Input: part model. Units: mm. Frame: model coordinates. A direction names the side the tool comes from. Round coordinates to 2 decimals unless told otherwise and drop trailing zeros. Loops run counter-clockwise (first coordinate to the right, second up) from the corner with the lowest first, then second, coordinate; pieces in that order, holes last. Notation, with made-up numbers: (49, 73) - (67, 73) arc R17 cw to (67, 87) - close; hole circle Ø10 at (72, 34). An arc over 180 degrees is marked (long way). One line per question, with ' | ' between items. Start each with the question number.
Item 1: Section A-A, the plane x = -47.5. Return loops of the section in (y, z).
Item 2: Set-up query: faces 1 (the face through (-31, 21, 0)), 2 (the face through (-31.04, 15.88, -10.9)), 3 (the face through (-31.04, -10.86, 15.84)), 4 (the face through (-31.035, 9.605, 9.713)), 5 (the face through (-42.5, 3, -3)). Return all of +Z, -Z, +X, -X, +Y, -Y with unobstructed straight access to the full face (end or side cutting, diameter ignored); none if empty.
Item 3: Section B-B, the plane x = 32. Return loops of the section in (y, z), plus the area to 3 significant figures.
Item 4: Material intervals for line 1 along Z through (x, y) = (-27.5, 0); line 2 along Z through (x, y) = (-33, 11.5); line 3 along X through (y, z) = (-11, 8), sorted ascending.
Item 5: First-contact query: pin 1 (9 mm diameter, centred on y = -11.5, z = -14, fed in from -X); pin 2 (1.3 mm diameter, centred on y = 17, z = 0, fed in from -X); pin 3 (1 mm diameter, centred on x = 2, y = 7.5, fed in from -Z). Flat tips, straight axial feed; report the tip coordinate or a pass-through.
Item 6: Draft query along Z for faces 6 (the face through (-33.5, -4.57, 12.35)), 7 (the face through (-23.57, -11.84, 14.364)), 8 (the face through (-28.246, -19.744, -6.218)). Return one class per face: pulls with the +Z half, pulls with the -Z half, needs draft (parallel to the pull), parting line crosses it, or undercut.
```python
from build123d import *

# Parameters (mm, degrees)
SKETCH1_W               = 0.5
SKETCH1_H               = 20.7
SKETCH1_W_2             = 23
SKETCH1_H_2             = 5
SKETCH2_R               = 2.1
CUT_EXTRUDE1_DEPTH      = 10
CUT_EXTRUDE2_DEPTH      = 16
CUT_EXTRUDE3_DEPTH      = 5
SKETCH14_R              = 2.25
CUT_EXTRUDE4_DEPTH      = 10
ENL_V_START             = -4
ESQUISSE4_R             = 4
ESQUISSE4_R_2           = 3
ENL_V_MAT_EXTRU_1_DEPTH = 4


with BuildPart() as part:
    # Sketch1 → Revolve3 (revolve)
    with BuildSketch(Plane.XY, mode=Mode.PRIVATE) as revolve3_sk:
        with BuildLine():
            Line((0, 20), (0, 0))
            Line((0, 0), (59.6, 0))
            Line((59.6, 0), (59.6, 8.75))
            Line((59.6, 8.75), (59.6, 21))
            Line((59.6, 21), (1, 21))
            ThreePointArc((1, 21), (0.292893219, 20.707106781), (0, 20))
        make_face()
        Polygon((-5, 0), (0, 0), (0, 20), (0, 21), (-5, 21), (-5, 20.7), align=None)
        with BuildLine():
            Line((59.6, 8.75), (59.6, 0))
            Line((59.6, 0), (62.6, 0))
            Line((62.6, 0), (62.6, 7.75))
            ThreePointArc((62.6, 7.75), (62.307106781, 8.457106781), (61.6, 8.75))
            Line((61.6, 8.75), (59.6, 8.75))
        make_face()
        with Locations((-5.25, 10.35)):
            Rectangle(SKETCH1_W, SKETCH1_H)
        with BuildLine():
            Line((62.6, 7.75), (62.6, 0))
            Line((62.6, 0), (63.6, 0))
            Line((63.6, 0), (63.6, 3))
            Line((63.6, 3), (63.6, 7.25))
            ThreePointArc((63.6, 7.25), (63.453553391, 7.603553391), (63.1, 7.75))
            Line((63.1, 7.75), (62.6, 7.75))
        make_face()
        Polygon((-28, 0), (-5.5, 0), (-5.5, 20.7), (-5.5, 21), (-28, 21), (-28, 20.7), align=None)
        with BuildLine():
            Line((63.6, 3), (63.6, 0))
            Line((63.6, 0), (65.6, 0))
            Line((65.6, 0), (65.6, 2.5))
            ThreePointArc((65.6, 2.5), (65.453553391, 2.853553391), (65.1, 3))
            Line((65.1, 3), (63.6, 3))
        make_face()
        with Locations((-28.25, 10.35)):
            Rectangle(SKETCH1_W, SKETCH1_H)
        Polygon((-33.5, 0), (-28.5, 0), (-28.5, 20.7), (-28.5, 21), (-33.5, 21), (-33.5, 13), align=None)
        Polygon((-35.5, 0), (-33.5, 0), (-33.5, 13), (-35.5, 13), (-35.5, 5), align=None)
        with Locations((-47, 2.5)):
            Rectangle(SKETCH1_W_2, SKETCH1_H_2)
    revolve(revolve3_sk.sketch.rotate(Axis((-106.294937031, 0, 0), (1, 0, 0)), 180), axis=Axis((-106.294937031, 0, 0), (1, 0, 0)))

    # Sketch2 → Cut-Extrude1 (cut)
    with BuildSketch(Plane.ZY.offset(33.5)):
        with Locations(Location((0, 17.5, 0), (0, 0, 270))):
            Circle(SKETCH2_R)
        with Locations(Location((17.5, 0, 0), (0, 0, 270))):
            Circle(SKETCH2_R)
        with Locations(Location((0, -17.5, 0), (0, 0, 270))):
            Circle(SKETCH2_R)
        with Locations(Location((-17.5, 0, 0), (0, 0, 270))):
            Circle(SKETCH2_R)
    extrude(amount=-CUT_EXTRUDE1_DEPTH, mode=Mode.SUBTRACT)

    # Sketch5 → Cut-Extrude2 (cut)
    with BuildSketch(Plane.ZY.offset(58.5)):
        Polygon((-4.949747468, 0.707106781), (-0.707106781, 4.949747468), (-1.414213562, 5.656854249), (-5.656854249, 1.414213562), align=None)
    extrude(amount=-CUT_EXTRUDE2_DEPTH, mode=Mode.SUBTRACT)

    # Sketch12 → Cut-Extrude3 (cut)
    with BuildSketch(Plane.ZY.offset(33.5)):
        with BuildLine():
            Line((9.629672349, 14.579093037), (12.132820594, 17.140439447))
            ThreePointArc((12.132820594, 17.140439447), (14.849242405, 14.849242405), (17.140439447, 12.132820594))
            Line((17.140439447, 12.132820594), (14.579093037, 9.629672349))
            ThreePointArc((14.579093037, 9.629672349), (9.65794686, 9.65794686), (9.629672349, 14.579093037))
        make_face()
        with BuildLine():
            Line((14.579093037, -9.629672349), (17.140439447, -12.132820594))
            ThreePointArc((17.140439447, -12.132820594), (14.849242405, -14.849242405), (12.132820594, -17.140439447))
            Line((12.132820594, -17.140439447), (9.629672349, -14.579093037))
            ThreePointArc((9.629672349, -14.579093037), (9.65794686, -9.65794686), (14.579093037, -9.629672349))
        make_face()
        with BuildLine():
            Line((-9.629672349, -14.579093037), (-12.132820594, -17.140439447))
            ThreePointArc((-12.132820594, -17.140439447), (-14.849242405, -14.849242405), (-17.140439447, -12.132820594))
            Line((-17.140439447, -12.132820594), (-14.579093037, -9.629672349))
            ThreePointArc((-14.579093037, -9.629672349), (-9.65794686, -9.65794686), (-9.629672349, -14.579093037))
        make_face()
        with BuildLine():
            Line((-14.579093037, 9.629672349), (-17.140439447, 12.132820594))
            ThreePointArc((-17.140439447, 12.132820594), (-14.849242405, 14.849242405), (-12.132820594, 17.140439447))
            Line((-12.132820594, 17.140439447), (-9.629672349, 14.579093037))
            ThreePointArc((-9.629672349, 14.579093037), (-9.65794686, 9.65794686), (-14.579093037, 9.629672349))
        make_face()
    extrude(amount=-CUT_EXTRUDE3_DEPTH, mode=Mode.SUBTRACT)

    # Sketch14 → Cut-Extrude4 (cut)
    with BuildSketch(Plane.ZY.offset(28.5)):
        with Locations(Location((12.132820594, 12.132820594, 0), (0, 0, 270))):
            Circle(SKETCH14_R)
        with Locations(Location((12.132820594, -12.132820594, 0), (0, 0, 270))):
            Circle(SKETCH14_R)
        with Locations(Location((-12.132820594, -12.132820594, 0), (0, 0, 270))):
            Circle(SKETCH14_R)
        with Locations(Location((-12.132820594, 12.132820594, 0), (0, 0, 270))):
            Circle(SKETCH14_R)
    extrude(amount=-CUT_EXTRUDE4_DEPTH, mode=Mode.SUBTRACT)

    # Esquisse4 → Enlèv. mat.-Extru.1 (cut)
    with BuildSketch(Plane(origin=(63.6, 0, 0), x_dir=(0, 0, -1), z_dir=(1, 0, 0)).offset(ENL_V_START)):
        with Locations(Location((0, 0, 0), (0, 0, 90))):
            Circle(ESQUISSE4_R)
        with Locations(Location((0, 0, 0), (0, 0, 270))):
            Circle(ESQUISSE4_R_2, mode=Mode.SUBTRACT)
    extrude(amount=ENL_V_MAT_EXTRU_1_DEPTH, mode=Mode.SUBTRACT)


solid = part.part
```
Return value:
1) outline: (0.71, -4.95) - (4.95, -0.71) arc R5 ccw (long way) to start
2) face 1: +X, -X, +Y | face 2: -Z, -X | face 3: -X, -Y | face 4: -X | face 5: -Z, -X, +Y
3) outline: circle Ø42 at (0, 0) | area: 1,390 mm2
4) line 1: -21 to -19.6, -15.4 to 15.4, 19.6 to 21 | line 2: -17.57 to -16.49, -8.69 to 8.69, 16.49 to 17.57 | line 3: -33.5 to 59.6
5) pin 1: x = -33.5 | pin 2: x = -23.5 | pin 3: z = -19.8
6) face 6: needs draft | face 7: undercut | face 8: parting line crosses it
